Check sheet for the modelled part. Datum: model origin and axes. Units: mm. A direction names the side the tool comes from. Round coordinates to 2 decimals unless told otherwise and drop trailing zeros. Write each loop counter-clockwise with the first axis right and the second up, starting at its lowest first coordinate (ties: lowest second). Pieces come first, ordered by that corner, then holes. Notation, with made-up numbers: M 34.5,31.25 L 40.5,31.25 A14 ccw 40.5,41.25 Z; hole C 10.5,65 d2. An arc over 180 degrees is marked long. One line per item, written item: value.
from build123d import *

# Parameters (mm, degrees)
MODEL_R             = 2.5
MODEL_R_2           = 2
MODEL_R_3           = 1.6
BOSS_EXTRUDE1_DEPTH = 3.2
SKETCH1_R           = 1.5005
CUT_EXTRUDE1_DEPTH  = 85.084719183


with BuildPart() as part:
    # Model → Boss-Extrude1 (new body)
    with BuildSketch(Plane.XY):
        Polygon((15.75, 55), (15.75, 45), (10.25, 45), (10.25, 55), (11.4, 55), (11.4, 62), (-20.35, 62), (-20.35, 55), (-19.2, 55), (-19.2, 45), (-24.7, 45), (-24.7, 55), (-23.55, 55), (-23.55, 62), (-31, 62), (-31, 66), (-52, 66), (-52, -66), (-31, -66), (-31, -62), (-23.55, -62), (-23.55, -55), (-24.7, -55), (-24.7, -45), (-19.2, -45), (-19.2, -55), (-20.35, -55), (-20.35, -62), (11.4, -62), (11.4, -55), (10.25, -55), (10.25, -45), (15.75, -45), (15.75, -55), (14.6, -55), (14.6, -62), (22, -62), (22, -66), (43, -66), (43, 66), (22, 66), (22, 62), (14.6, 62), (14.6, 55), align=None)
        with Locations((-42, -4)):
            Circle(MODEL_R, mode=Mode.SUBTRACT)
        with Locations((-42, 58)):
            Circle(MODEL_R, mode=Mode.SUBTRACT)
        with Locations((35, 50)):
            Circle(MODEL_R, mode=Mode.SUBTRACT)
        with Locations((35, -4)):
            Circle(MODEL_R, mode=Mode.SUBTRACT)
        with Locations((35, 58)):
            Circle(MODEL_R, mode=Mode.SUBTRACT)
        with Locations((35, 4)):
            Circle(MODEL_R, mode=Mode.SUBTRACT)
        with Locations((-42, 4)):
            Circle(MODEL_R, mode=Mode.SUBTRACT)
        with Locations((-42, 50)):
            Circle(MODEL_R, mode=Mode.SUBTRACT)
        with Locations((-20, -35)):
            Circle(MODEL_R_2, mode=Mode.SUBTRACT)
        with Locations((10, -35)):
            Circle(MODEL_R_2, mode=Mode.SUBTRACT)
        with Locations((10, -11)):
            Circle(MODEL_R_3, mode=Mode.SUBTRACT)
        with Locations((25, -11)):
            Circle(MODEL_R_3, mode=Mode.SUBTRACT)
        with Locations((-5, 57)):
            Circle(MODEL_R_3, mode=Mode.SUBTRACT)
        with Locations((-5, -57)):
            Circle(MODEL_R_3, mode=Mode.SUBTRACT)
        with Locations((-35, -11)):
            Circle(MODEL_R_3, mode=Mode.SUBTRACT)
        with Locations((-20, -11)):
            Circle(MODEL_R_3, mode=Mode.SUBTRACT)
        with Locations((-5, -11)):
            Circle(MODEL_R_3, mode=Mode.SUBTRACT)
    extrude(amount=BOSS_EXTRUDE1_DEPTH)

    # Sketch1 → Cut-Extrude1 (cut, through all)
    with BuildSketch(Plane.XY.offset(3.2)):
        with Locations((-29.4995, 62)):
            Circle(SKETCH1_R)
        with Locations((20.4995, 62)):
            Circle(SKETCH1_R)
        with Locations((20.4995, -62)):
            Circle(SKETCH1_R)
        with Locations((-29.4995, -62)):
            Circle(SKETCH1_R)
    extrude(amount=-CUT_EXTRUDE1_DEPTH, mode=Mode.SUBTRACT)


solid = part.part
Q1. Access from +Z, -Z, +X, -X, +Y, -Y to the whole of each face (thin tool, end or side, straight path). Record for faces 3 (the flat face through (-42, -66, 2)), 4 (the flat face through (-22, -45, 2)), 5 (the flat face through (-20.35, -58, 2)), 6 (the flat face through (14.6, 59, 2)).
Completed:
face 3: +Z, -Z, +X, -X, -Y
face 4: +Z, -Z
face 5: +Z, -Z, -Y
face 6: +Z, -Z, +Y
Q2. Sectioned sample at B-B on x = -35. Enter the section's corners in (y, z).
Completed:
outline: M -66,0 L -12.6,0 L -12.6,3.2 L -66,3.2 Z; M -9.4,0 L 66,0 L 66,3.2 L -9.4,3.2 Z
Q3. Draft check along X on faces 1 (the cylindrical face through (-6.6, 57.07, 1.58)), 2 (the flat face through (-41, 66, 2)). Enter one of: pulls with the +X half, pulls with the -X half, needs draft (parallel to the pull), parting line crosses it, or undercut.
Completed:
face 1: undercut
face 2: needs draft
Q4. Sectioned sample at A-A on y = -35. Enter the section's corners in (x, z), and give its area (3 significant figures).
Completed:
outline: M -52,0 L -22,0 L -22,3.2 L -52,3.2 Z; M -18,0 L 8,0 L 8,3.2 L -18,3.2 Z; M 12,0 L 43,0 L 43,3.2 L 12,3.2 Z
area: 278 mm^2
Q5. Sectioned sample at C-C on y = 4. Enter the section's corners in (x, z), and give its area (3 significant figures).
Completed:
outline: M -52,0 L -44.5,0 L -44.5,3.2 L -52,3.2 Z; M -39.5,0 L 32.5,0 L 32.5,3.2 L -39.5,3.2 Z; M 37.5,0 L 43,0 L 43,3.2 L 37.5,3.2 Z
area: 272 mm^2
Q6. Scan lines: line 1 (Y direction, x = -42, z = 2.5); line 2 (Y direction, x = -5, z = 0.9); line 3 (X direction, y = -52.5, z = 0.4). Record each from-to range of solid material in increasing order. Write a range as [from, to].
Completed:
line 1: [-66, -6.5], [-1.5, 1.5], [6.5, 47.5], [52.5, 55.5], [60.5, 66]
line 2: [-62, -58.6], [-55.4, -12.6], [-9.4, 55.4], [58.6, 62]
line 3: [-52, -24.7], [-19.2, 10.25], [15.75, 43]
Q7. Depth check by flat-ended pin: P1, Ø3, axis at x = -5, y = -11, coming from the -Z side; P2, Ø1, axis at x = -21, z = 1, coming from the -Y side; P3, Ø1, axis at x = 16, z = 1.5, coming from the +Y side; P4, Ø0.9, axis at x = 15.5, z = 1.5, coming from the -Y side. Enter the tip coordinate at first touch or a pass-through.
Completed:
P1: through
P2: y = -45
P3: y = 62
P4: y = -62
Q8. Sectioned sample at D-D on z = 1.05. State how many separate pieces and enclosed holes the cut face has, and give its area (3 significant figures).
Completed:
separate pieces: 1
enclosed holes: 17
area: 11,600 mm^2
